Build history of the part. All positions in model axes, mm. Face numbers are marked on the shaded views. A direction names the side the tool comes from. Give positions to 0.01 mm unless a question says otherwise; leave off trailing zeros. Order: outer loops, then holes, each group sorted by start corner. A loop starts at its lowest first (then second) coordinate and runs counter-clockwise, first axis right, second up. Notation, with made-up numbers: M 63.25,30 L 90.25,30 A21 cw 90.25,38 Z; hole C 20.5,45.5 d2. An arc over 180 degrees is marked long. One line per item, written item: value.
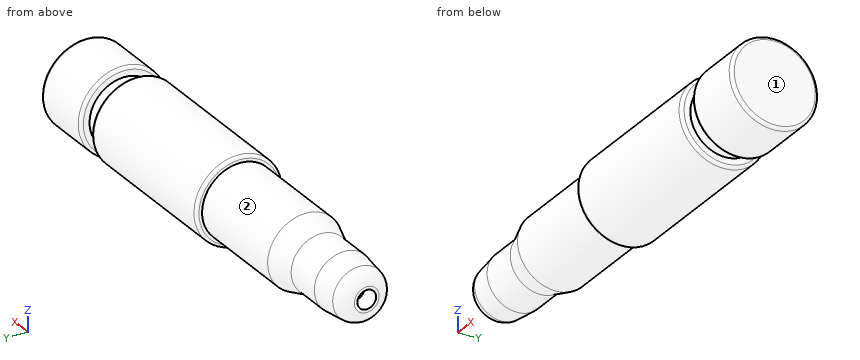
from build123d import *

# Parameters (mm, degrees)
ESBO_O2_R             = 1.5
CORTE_EXTRUS_O1_DEPTH = 3
FILETE1_R             = 2.25
FILETE2_R             = 0.5


with BuildPart() as part:
    # Esboço1 → Revolução1 (revolve)
    with BuildSketch(Plane.XY, mode=Mode.PRIVATE) as revolu_o1_sk:
        Polygon((0, 0), (73, 0), (73, 7), (63, 7), (63, 5.5), (60, 5.5), (60, 7), (33, 7), (33, 6), (16, 6), (12, 4.7), (6, 4.7), (0, 4), align=None)
    revolve(revolu_o1_sk.sketch.rotate(Axis((0, 0, 0), (1, 0, 0)), 90), axis=Axis((0, 0, 0), (1, 0, 0)))

    # Esboço2 → Corte-extrusão1 (cut)
    with BuildSketch(Plane.ZY):
        Circle(ESBO_O2_R)
    extrude(amount=-CORTE_EXTRUS_O1_DEPTH, mode=Mode.SUBTRACT)

    # Filete1
    filete1_edges = [part.edges().sort_by_distance(p)[0] for p in [
        (0, 0, -4),
    ]]
    fillet(filete1_edges, radius=FILETE1_R)

    # Filete2
    filete2_edges = [part.edges().sort_by_distance(p)[0] for p in [
        (33, 0, -7),
        (60, 0, -7),
        (63, 0, -7),
        (73, 0, -7),
    ]]
    fillet(filete2_edges, radius=FILETE2_R)


solid = part.part
1) Drill centre lines: probe 1 along X at (y, z) = (-5, -4.25); probe 2 along Y at (x, z) = (2.25, 0); probe 3 along Z at (x, y) = (12, 4.25). Where is each one in solid material? Low to high. Write a range as from..to.
Check values:
probe 1: 33..60, 63..73
probe 2: -4.26..-1.5, 1.5..4.26
probe 3: -2.01..2.01
2) Saw through at A-A, the plane x = 39. Write the cut outline in (y, z), then the cut area to 3 significant figures.
Check values:
outline: C 0,0 d14
area: 154 mm^2
3) Pin check, flat tips, straight feed: pin 1 (1 mm diameter, centred on x = 40, z = -4.5, fed in from -Y); pin 2 (8 mm diameter, centred on x = 23.5, y = -1, fed in from -Z); pin 3 (4 mm diameter, centred on x = 53.5, z = 5, fed in from +Y). Stop position of each tip, or through.
Check values:
pin 1: y = -5.74
pin 2: z = -6
pin 3: y = 6.32
4) Tool access for the marked faces 1 and 2: list every direction of +Z, -Z, +X, -X, +Y, -Y with a clear straight run to the whole face (end or side of a thin tool).
Check values:
face 1: +Z, -Z, +X, +Y, -Y
face 2: -X
5) Saw through at B-B, the plane x = 25. Write the cut outline in (y, z), then the cut area to 3 significant figures.
Check values:
outline: C 0,0 d12
area: 113 mm^2
